from build123d import *

# Parameters (mm, degrees)
BOSS_EXTRUDE1_DEPTH = 30


with BuildPart() as part:
    # Sketch1 → Boss-Extrude1 (new body)
    with BuildSketch(Plane.XY):
        with BuildLine():
            Line((-2.5, 1.5), (-1.5, 1.5))
            Line((-1.5, 1.5), (-1.5, 2.5))
            ThreePointArc((-1.5, 2.5), (0, 4), (1.5, 2.5))
            Line((1.5, 2.5), (1.5, 1.5))
            Line((1.5, 1.5), (2.5, 1.5))
            ThreePointArc((2.5, 1.5), (4, 0), (2.5, -1.5))
            Line((2.5, -1.5), (1.5, -1.5))
            Line((1.5, -1.5), (1.5, -2.5))
            ThreePointArc((1.5, -2.5), (0, -4), (-1.5, -2.5))
            Line((-1.5, -2.5), (-1.5, -1.5))
            Line((-1.5, -1.5), (-2.5, -1.5))
            ThreePointArc((-2.5, -1.5), (-4, 0), (-2.5, 1.5))
        make_face()
    extrude(amount=BOSS_EXTRUDE1_DEPTH)


solid = part.part
Read the model definition and answer for the solid it produces. Units are mm, in the model's axes. A direction names the side the tool comes from. Coordinates: 2 decimals unless noted, no trailing zeros. Write each loop counter-clockwise with the first axis right and the second up, starting at its lowest first coordinate (ties: lowest second). Pieces come first, ordered by that corner, then holes. Notation, with made-up numbers: M -8,-9.75 L 14,-9.75 A19 cw 14,13.25 Z; hole C 15,86.5 d10. An arc over 180 degrees is marked long. Use a Markdown table: item, result.
Q1. The part is cut by section C-C, the plane x = -3. Write down the section's boundary in (y, z), then the cut area to 3 significant figures.
Answer block:
| item | result |
|---|---|
| outline | M -1.41,0 L 1.41,0 L 1.41,30 L -1.41,30 Z |
| area | 84.9 mm2 |
Q2. Straight lines are drawn through the part: L1, parallel to Y at x = -2.5, z = 20.25; L2, parallel to X at y = -0.25, z = 22.5. For each, find the intervals that lie inside material, in ascending order. Write a range as [from, to].
Answer block:
| item | result |
|---|---|
| L1 | y = [-1.5, 1.5] |
| L2 | x = [-3.98, 3.98] |
Q3. The part is cut by section B-B, the plane y = 0.5. Write down the section's boundary in (x, z), then the cut area to 3 significant figures.
Answer block:
| item | result |
|---|---|
| outline | M -3.91,0 L 3.91,0 L 3.91,30 L -3.91,30 Z |
| area | 235 mm2 |
Q4. Each of these flat-tipped pins is pushed along its axis until it touches: pin 1 Ø3 at (x, z) = (-2, 8.5) entering from -Y; pin 2 Ø0.5 at (x, z) = (2, 8) entering from +Y; pin 3 Ø2 at (x, y) = (-3, 3) entering from +Z; pin 4 Ø0.8 at (y, z) = (2, 14.5) entering from -X. Where does it stop, or does it pass through?
Answer block:
| item | result |
|---|---|
| pin 1 | stops at y = -3.91 |
| pin 2 | stops at y = 1.5 |
| pin 3 | passes through |
| pin 4 | stops at x = -1.5 |
Q5. The part is cut by section A-A, the plane z = 16.25. Write down the section's boundary in (x, y).
Answer block:
| item | result |
|---|---|
| outline | M -2.5,-1.5 L -1.5,-1.5 L -1.5,-2.5 A1.5 ccw 1.5,-2.5 L 1.5,-1.5 L 2.5,-1.5 A1.5 ccw 2.5,1.5 L 1.5,1.5 L 1.5,2.5 A1.5 ccw -1.5,2.5 L -1.5,1.5 L -2.5,1.5 A1.5 ccw Z |
Q6. Which of the six approach directions +Z, -Z, +X, -X, +Y, -Y give full straight-line access (tool end or side, diameter ignored) to faces 1 (the face through (-2, -1.5, 15)), 2 (the face through (1.5, 2, 15)), 3 (the face through (-2, 1.5, 15))?
Answer block:
| item | result |
|---|---|
| face 1 | +Z, -Z, -X, -Y |
| face 2 | +Z, -Z, +X, +Y |
| face 3 | +Z, -Z, -X, +Y |
